```python
from build123d import *

# Parameters (mm, degrees)
SKETCH1_R           = 1
BOSS_EXTRUDE1_DEPTH = 12
SKETCH2_R           = 1.75
BOSS_EXTRUDE2_DEPTH = 1.3
BOSS_EXTRUDE2_TAPER = 32
SKETCH3_W           = 0.5
SKETCH3_H           = 1.258378485
SKETCH3_H_2         = 1.241621515
SKETCH3_W_2         = 1.234727157
SKETCH3_H_3         = 0.5
SKETCH3_W_3         = 1.265272843
CUT_EXTRUDE1_DEPTH  = 0.3


with BuildPart() as part:
    # Sketch1 → Boss-Extrude1 (new body)
    with BuildSketch(Plane(origin=(0, 0, 0), x_dir=(1, 0, 0), z_dir=(0, 1, 0))):
        Circle(SKETCH1_R)
    extrude(amount=BOSS_EXTRUDE1_DEPTH)

    # Sketch2 → Boss-Extrude2 (add)
    with BuildSketch(Plane(origin=(0, 12, 0), x_dir=(1, 0, 0), z_dir=(0, 1, 0))):
        Circle(SKETCH2_R)
    extrude(amount=-BOSS_EXTRUDE2_DEPTH, taper=BOSS_EXTRUDE2_TAPER)

    # Sketch3 → Cut-Extrude1 (cut)
    with BuildSketch(Plane(origin=(0, 12, 0), x_dir=(1, 0, 0), z_dir=(0, 1, 0))):
        with Locations((-0.015272843, 0.870810758)):
            Rectangle(SKETCH3_W, SKETCH3_H)
        with Locations((-0.015272843, -0.879189242)):
            Rectangle(SKETCH3_W, SKETCH3_H_2)
        with Locations((-0.882636421, -0.008378485)):
            Rectangle(SKETCH3_W_2, SKETCH3_H_3)
        with Locations((0.867363579, -0.008378485)):
            Rectangle(SKETCH3_W_3, SKETCH3_H_3)
        with Locations((-0.015272843, -0.008378485)):
            Rectangle(SKETCH3_W, SKETCH3_H_3)
    extrude(amount=-CUT_EXTRUDE1_DEPTH, mode=Mode.SUBTRACT)


solid = part.part
```
Read the model definition and answer for the solid it produces. Units are mm, in the model's axes. Give positions to 0.01 mm unless a question says otherwise; leave off trailing zeros. Loops run counter-clockwise (first coordinate to the right, second up) from the corner with the lowest first, then second, coordinate; pieces in that order, holes last.
Item 1: Find the intervals of material crossed by line 1 along Z through (x, y) = (0, 4.5); line 2 along Y through (x, z) = (-0.9, -0.05); line 3 along X through (y, z) = (0.75, 0.8), in increasing order.
Item 2: The part is cut by section A-A (x = 0). Write down the section's boundary in (y, z), and give its area (3 significant figures).
Item 3: The part is cut by section B-B (y = 3.5). Write down the section's boundary in (x, z).
Item 4: The mould has two halves that part along X. Classify faces 1 (the cylindrical face through (0, 5, 1)), 2 (the flat face through (0.4, 12, -0.4)), 3 (the flat face through (0, 11.7, 0)): released by +X, released by -X, zero draft, split by the parting line, or undercut.
Taken from the geometry:
1. line 1: z = -1 to 1
1. line 2: y = 0 to 11.7
1. line 3: x = -0.6 to 0.6
2. outline: (0, -1) - (10.8, -1) - (12, -1.75) - (12, -1.5) - (11.7, -1.5) - (11.7, 1.5) - (12, 1.5) - (12, 1.75) - (10.8, 1) - (0, 1) - close
2. area: 24.0 mm2
3. outline: circle Ø2 at (0, 0)
4. face 1: split by the parting line
4. face 2: zero draft
4. face 3: undercut
